Build history of the part. All positions in model axes, mm. Face numbers are marked on the shaded views. A direction names the side the tool comes from. Coordinates: 2 decimals unless noted, no trailing zeros. Order: outer loops, then holes, each group sorted by start corner. A loop starts at its lowest first (then second) coordinate and runs counter-clockwise, first axis right, second up. Notation, with made-up numbers: M 54.5,63 L 108.5,63 A16 cw 108.5,79 Z; hole C -13,-5.5 d5. An arc over 180 degrees is marked long. Write item = value, one per line. Start each with the question number.
Q1. Band-saw the part on D-D on z = 0.5. Write the cut outline in (x, y), plus the area to 3 significant figures.
Q2. 3-axis set-ups, long thin cutter, end or side, ignore diameter. For the marked faces 1, 2 and 3: which of +Z, -Z, +X, -X, +Y, -Y reach the whole face in a straight line?
Q3. Pin check, flat tips, straight feed: P1, Ø1, axis at x = -4.5, y = -5, coming from the -Z side; P2, Ø1.5, axis at y = 3, z = -3, coming from the +X side; P3, Ø1.5, axis at y = 2.5, z = -1.5, coming from the +X side. Stop position of each tip, or through.
Q4. Pull direction X, two halves, no side cores. Call the marked faces 4, 5 and 6: released by +X, released by -X, zero draft, split by the parting line, or undercut.
Q5. Band-saw the part on A-A on x = 0. Write the cut outline in (y, z).
Q6. Drill centre lines: probe 1 along Y at (x, z) = (0, 3.9); probe 2 along Z at (x, y) = (5.5, 0.5); probe 3 along Z at (x, y) = (3.5, 1). Where is each one in solid material? Low to high.
Q7. Band-saw the part on C-C on z = 3.75. Write the cut outline in (x, y), plus the area to 3 significant figures.
```python
from build123d import *

# Parameters (mm, degrees)
SZKIC1_R                    = 7.5
DODANIE_WYCI_GNI_CIE1_DEPTH = 3
SZKIC2_R                    = 3.8
DODANIE_WYCI_GNI_CIE2_DEPTH = 4
SZKIC3_R                    = 7.5
SZKIC3_R_2                  = 4.25
DODANIE_WYCI_GNI_CIE3_DEPTH = 1.8


with BuildPart() as part:
    # Szkic1 → Dodanie-wyciągnięcie1 (new body)
    with BuildSketch(Plane.XY):
        Circle(SZKIC1_R)
    extrude(amount=DODANIE_WYCI_GNI_CIE1_DEPTH)

    # Szkic2 → Dodanie-wyciągnięcie2 (add)
    with BuildSketch(Plane(origin=(0, 0, 0), x_dir=(-1, 0, 0), z_dir=(0, 0, -1))):
        Circle(SZKIC2_R)
    extrude(amount=DODANIE_WYCI_GNI_CIE2_DEPTH)

    # Szkic3 → Dodanie-wyciągnięcie3 (add)
    with BuildSketch(Plane.XY.offset(3)):
        Circle(SZKIC3_R)
        Circle(SZKIC3_R_2, mode=Mode.SUBTRACT)
    extrude(amount=DODANIE_WYCI_GNI_CIE3_DEPTH)


solid = part.part
```
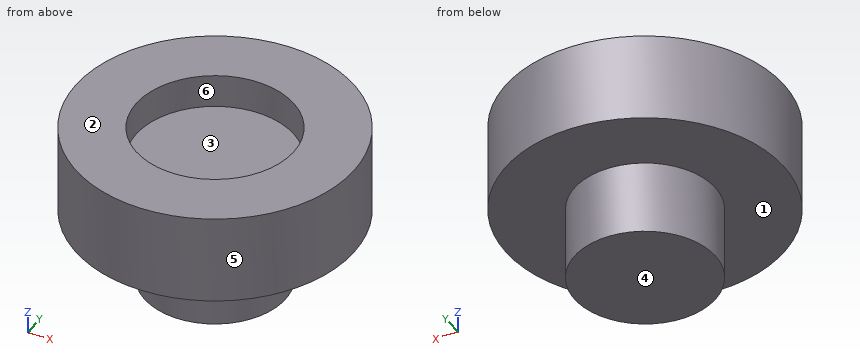
Recorded:
q1.outline = C 0,0 d15
q1.area = 177 mm2
q2.face_1 = -Z
q2.face_2 = +Z, +X, -X, +Y, -Y
q2.face_3 = +Z
q3.P1 = 0
q3.P2 = 3.06
q3.P3 = 3.37
q4.face_4 = zero draft
q4.face_5 = split by the parting line
q4.face_6 = undercut
q5.outline = M -7.5,0 L -3.8,0 L -3.8,-4 L 3.8,-4 L 3.8,0 L 7.5,0 L 7.5,4.8 L 4.25,4.8 L 4.25,3 L -4.25,3 L -4.25,4.8 L -7.5,4.8 Z
q6.probe_1 = -7.5 to -4.25, 4.25 to 7.5
q6.probe_2 = 0 to 4.8
q6.probe_3 = -4 to 3
q7.outline = C 0,0 d15; hole C 0,0 d8.5
q7.area = 120 mm2
